from build123d import *

# Parameters (mm, degrees)
SM_BASE_FLANGE_1_DEPTH      = 10
SM_EDGE_FLANGE_2_DEPTH      = 18
SM_START                    = 1
SM_EDGE_FLANGE_2_FLAT_DEPTH = 1


# Sheet-metal steps are written as plain solids
with BuildPart() as part:
    # Sketch 1 → 基体-法兰1 (new body)
    with BuildSketch(Plane.XY):
        with BuildLine():
            Line((0, 0), (18, 0))
            ThreePointArc((18, 0), (19.414213562, 0.585786438), (20, 2))
            Line((20, 2), (20, 15))
            Line((20, 15), (21, 15))
            Line((21, 15), (21, 2))
            ThreePointArc((21, 2), (20.121320344, -0.121320344), (18, -1))
            Line((18, -1), (0, -1))
            Line((0, -1), (0, 0))
        make_face()
    extrude(amount=SM_BASE_FLANGE_1_DEPTH)

    # 边线-法兰2 bend section (across the edge) → 边线-法兰2 (add)
    with BuildSketch(Plane(origin=(18, -1, 13), x_dir=(0, 0, -1), z_dir=(-1, 0, 0))):
        with BuildLine():
            Line((-1, 3), (0, 3))
            ThreePointArc((0, 3), (0.878679656, 0.878679656), (3, 0))
            Line((3, 0), (3, -1))
            ThreePointArc((3, -1), (0.171572875, 0.171572875), (-1, 3))
        make_face()
    extrude(amount=SM_EDGE_FLANGE_2_DEPTH)

    # 边线-法兰2 profile (on flange) → 边线-法兰2 flat (add)
    with BuildSketch(Plane(origin=(0, -1, 13), x_dir=(-1, 0, 0), z_dir=(0, 0, 1)).offset(SM_START)):
        Polygon((0, 3), (0, 10), (-1.8, 12.5), (-16.2, 12.5), (-18, 10), (-18, 3), align=None)
    extrude(amount=-SM_EDGE_FLANGE_2_FLAT_DEPTH)


solid = part.part
Geometry: final body of the model. Coordinates: model frame, mm. A direction names the side the tool comes from. Round coordinates to 2 decimals unless told otherwise and drop trailing zeros. Order: outer loops, then holes, each group sorted by start corner. A loop starts at its lowest first (then second) coordinate and runs counter-clockwise, first axis right, second up.
Q1. Material intervals for probe 1 along Z at (x, y) = (2.5, -7.5); probe 2 along X at (y, z) = (4, 4); probe 3 along Y at (x, z) = (6, 7.5), sorted ascending.
Result sheet:
probe 1: z = 13 to 14
probe 2: x = 20 to 21
probe 3: y = -1 to 0
Q2. Pin query (flat end, axial travel): pin 1 (8 mm diameter, centred on y = 11, z = 7, fed in from -X); pin 2 (5 mm diameter, centred on x = 12.5, z = 5.5, fed in from -Y); pin 3 (3 mm diameter, centred on x = 4.5, z = 6.5, fed in from +Y). Return the tip coordinate at first contact, or that it passes through.
Result sheet:
pin 1: stops at x = 20
pin 2: stops at y = -1
pin 3: stops at y = 0
Q3. Section B-B, the plane z = 4. Output: boundary loops of the cut face in (x, y), and give its area (3 significant figures).
Result sheet:
outline: (0, -1) - (18, -1) arc R3 ccw to (21, 2) - (21, 15) - (20, 15) - (20, 2) arc R2 cw to (18, 0) - (0, 0) - close
area: 34.9 mm2
Q4. Section D-D, the plane y = -2.75. Output: boundary loops of the cut face in (x, z), and give its area (3 significant figures).
Result sheet:
outline: (0, 12.73) - (18, 12.73) - (18, 13.8) - (0, 13.8) - close
area: 19.3 mm2
Q5. Section C-C, the plane y = 2.5. Output: boundary loops of the cut face in (x, z).
Result sheet:
outline: (20, 0) - (21, 0) - (21, 10) - (20, 10) - close
Q6. Access query for faces 1 (the face through (9, -9, 13)), 2 (the face through (8.9, -13.5, 13.5)), 3 (the face through (9, 0, 5)). Directions: +Z, -Z, +X, -X, +Y, -Y. A direction counts if a zero-diameter tool reaches every point of the face in a straight line with its end or side. Return the directions, or none.
Result sheet:
face 1: -Z, +X, -X, -Y
face 2: +Z, -Z, +X, -X, -Y
face 3: +Z, -Z, -X, +Y
Q7. Section A-A, the plane x = 8.75. Output: boundary loops of the cut face in (y, z), and give its area (3 significant figures).
Result sheet:
outline: (-13.5, 13) - (-4, 13) arc R3 cw to (-1, 10) - (-1, 0) - (0, 0) - (0, 10) arc R4 ccw to (-4, 14) - (-13.5, 14) - close
area: 25.0 mm2
